CAD build for the part. Positions are in the model's coordinates, mm. Coordinates: 2 decimals unless noted, no trailing zeros. Write each loop counter-clockwise with the first axis right and the second up, starting at its lowest first coordinate (ties: lowest second). Pieces come first, ordered by that corner, then holes. Notation, with made-up numbers: (28, 11.25) - (47, 11.25) arc R3 ccw to (47, 15.25) - close; hole circle Ø6 at (20, 66.25). An arc over 180 degrees is marked (long way). One line per question, with ' | ' between items. Start each with the question number.
1. Band-saw the part on B-B, the plane z = 7. Write the cut outline in (x, y).
2. Band-saw the part on A-A, the plane y = -300. Write the cut outline in (x, z), then the cut area to 3 significant figures.
3. Two-plate mould, pull along X, no slides. Class faces 1 (the flat face through (-28, -187.34, -7.86)), 2 (the flat face through (-46, 0, -16)), 3 (the cylindrical face through (56.62, -372.77, -164.07)): +X half, -X half, draft (parallel to the pull), parting line (faces both ways), or undercut.
4. Probe line 1 (Z direction, x = -18, y = -222); line 2 (Z direction, x = -130.5, y = -348); line 3 (X direction, y = -149.5, z = -124.5). List the from-to ranges inside material, lowest first.
5. Band-saw the part on C-C, the plane x = -145. Give the number of separate pieces and of enclosed holes in the cut face, then the cut area to 3 significant figures.
6. Flat gauge pins, fed straight in: P1, Ø10, axis at x = -96.5, y = -208, coming from the +Z side; P2, Ø4, axis at y = -106.5, z = -12.5, coming from the +X side; P3, Ø10, axis at x = -70.5, y = -315.5, coming from the -Z side. Where does each tip first touch, or does it go through?
from build123d import *

# Parameters (mm, degrees)
F1_DEPTH = 380
F2_R     = 3
F3_DEPTH = 40


with BuildPart() as f1:
    # F0 (on Front) → F1 (new body)
    with BuildSketch(Plane.XZ):
        Polygon((79.4555794589, -161.3228202568), (-138.5034663545, 149.954956573), (-171.269548126, 127.011899119), (46.6894976874, -184.2658777108), align=None)
    extrude(amount=F1_DEPTH)

    # F2 (on face) → F3 (cut, through all)
    with BuildSketch(Plane(origin=(-55.2475195846, 0, -38.6847296806), x_dir=(0, -1, 0), z_dir=(-0.8191520443, 0, -0.5735764364))):
        with Locations((370, 190.2782338819)):
            Circle(F2_R)
        with Locations((370, -165.7217661181)):
            Circle(F2_R)
        with Locations((10, -165.7217661181)):
            Circle(F2_R)
        with Locations((10, 190.2782338819)):
            Circle(F2_R)
    extrude(amount=-F3_DEPTH, mode=Mode.SUBTRACT)


solid = f1.part
Filled in:
1) outline: (-87.24, -380) - (-38.41, -380) - (-38.41, 0) - (-87.24, 0) - close
2) outline: (-171.27, 127.01) - (46.69, -184.27) - (79.46, -161.32) - (-138.5, 149.95) - close | area: 15,200 mm²
3) face 1: +X half | face 2: draft | face 3: undercut
4) line 1: z = -91.88 to -22.14 | line 2: z = 68.79 to 138.52 | line 3: x = 4.84 to 53.67
5) separate pieces: 1 | enclosed holes: 2 | area: 21,200 mm²
6) P1: stops at z = 97.11 | P2: stops at x = -23.35 | P3: stops at z = -24.04
